```python
from build123d import *

# Parameters (mm, degrees)
F0_W          = 28
F0_H          = 28
F1_DEPTH      = 384.5
F2_W          = 32
F2_H          = 32
F2_W_2        = 28
F2_H_2        = 28
F3_DEPTH      = 608
F3_DEPTH_BACK = 25
F4_W          = 99.2901008725
F4_H          = 100
F5_DEPTH      = 6
F6_R          = 41
F7_DEPTH      = 32.001


with BuildPart() as f1:
    # F0 (on Right) → F1 (new body, symmetric)
    with BuildSketch(Plane.YZ):
        with BuildLine():
            ThreePointArc((-335, -14), (-334.4142135624, -15.4142135624), (-333, -16))
            Line((-333, -16), (-305, -16))
            ThreePointArc((-305, -16), (-303.5857864376, -15.4142135624), (-303, -14))
            Line((-303, -14), (-303, 14))
            ThreePointArc((-303, 14), (-303.5857864376, 15.4142135624), (-305, 16))
            Line((-305, 16), (-333, 16))
            ThreePointArc((-333, 16), (-334.4142135624, 15.4142135624), (-335, 14))
            Line((-335, 14), (-335, -14))
        make_face()
        with Locations((-319, 0)):
            Rectangle(F0_W, F0_H, mode=Mode.SUBTRACT)
    extrude(amount=F1_DEPTH, both=True)



with BuildPart() as f1b:
    # F0 (on Right) → F1, piece 2 (new body, symmetric)
    with BuildSketch(Plane.YZ):
        with BuildLine():
            ThreePointArc((335, 14), (334.4142135624, 15.4142135624), (333, 16))
            Line((333, 16), (305, 16))
            ThreePointArc((305, 16), (303.5857864376, 15.4142135624), (303, 14))
            Line((303, 14), (303, -14))
            ThreePointArc((303, -14), (303.5857864376, -15.4142135624), (305, -16))
            Line((305, -16), (333, -16))
            ThreePointArc((333, -16), (334.4142135624, -15.4142135624), (335, -14))
            Line((335, -14), (335, 14))
        make_face()
        with Locations((319, 0)):
            Rectangle(F0_W, F0_H, mode=Mode.SUBTRACT)
    extrude(amount=F1_DEPTH, both=True)


with BuildPart() as f1_1:
    add(f1.part)

    add(f1b.part)  # F3 merges F1b
    # F2 (on face) → F3 (join, two sides)
    with BuildSketch(Plane(origin=(0, -303, 0), x_dir=(-1, 0, 0), z_dir=(0, 1, 0))) as f3_sk:
        with Locations((-65.2901008725, 0)):
            Rectangle(F2_W, F2_H)
        with Locations((-65.2901008725, 0)):
            Rectangle(F2_W_2, F2_H_2, mode=Mode.SUBTRACT)
        with Locations((65.2901008725, 0)):
            Rectangle(F2_W, F2_H)
        with Locations((65.2901008725, 0)):
            Rectangle(F2_W_2, F2_H_2, mode=Mode.SUBTRACT)
    extrude(amount=F3_DEPTH)
    extrude(f3_sk.sketch, amount=-F3_DEPTH_BACK)

    # F4 (on face) → F5 (join)
    with BuildSketch(Plane.XY.offset(16)):
        with Locations((0.3549495637, 0)):
            Rectangle(F4_W, F4_H)
    extrude(amount=-F5_DEPTH)

    # F6 (on face) → F7 (cut, through all)
    with BuildSketch(Plane.XY.offset(16)):
        Circle(F6_R)
    extrude(amount=-F7_DEPTH, mode=Mode.SUBTRACT)


solid = f1_1.part
```
Input: part model. Units: mm. Frame: model coordinates. A direction names the side the tool comes from. Round coordinates to 2 decimals unless told otherwise and drop trailing zeros. Write each loop counter-clockwise with the first axis right and the second up, starting at its lowest first coordinate (ties: lowest second). Pieces come first, ordered by that corner, then holes. Notation, with made-up numbers: (-34, 18) - (13, 18) arc R20 cw to (13, 47) - close; hole circle Ø7 at (43.25, 3). An arc over 180 degrees is marked (long way). Write item = value, one per line.
(1) Section query B-B on x = -191.5. Output: boundary loops of the cut face in (y, z).
Geometry check:
outline = (-335, -14) arc R2 ccw to (-333, -16) - (-305, -16) arc R2 ccw to (-303, -14) - (-303, 14) arc R2 ccw to (-305, 16) - (-333, 16) arc R2 ccw to (-335, 14) - close; (303, -14) arc R2 ccw to (305, -16) - (333, -16) arc R2 ccw to (335, -14) - (335, 14) arc R2 ccw to (333, 16) - (305, 16) arc R2 ccw to (303, 14) - close; hole (-333, -14) - (-305, -14) - (-305, 14) - (-333, 14) - close; hole (305, -14) - (333, -14) - (333, 14) - (305, 14) - close
(2) Access query for faces 1 (the flat face through (1, 303, 0)), 2 (the flat face through (81.29, -316, 0)), 3 (the flat face through (51.29, -4, 0)), 4 (the flat face through (5, 319, -14)). Directions: +Z, -Z, +X, -X, +Y, -Y. A direction counts if a zero-diameter tool reaches every point of the face in a straight line with its end or side. Return the directions, or none.
Geometry check:
face_1 = +Z, -Z
face_2 = +X
face_3 = none
face_4 = +X, -X
(3) Section query C-C on x = 0. State how many separate pieces and enclosed holes the cut face has, then the cut area to 3 significant figures.
Geometry check:
separate_pieces = 4
enclosed_holes = 2
area = 581 mm^2
(4) Material intervals for probe 1 along X at (y, z) = (-117, 11.5); probe 2 along Y at (x, z) = (227, 1.5); probe 3 along Y at (x, z) = (0, 11.65), sorted ascending.
Geometry check:
probe_1 = -81.29 to -79.29, -51.29 to -49.29, 49.29 to 51.29, 79.29 to 81.29
probe_2 = -335 to -333, -305 to -303, 303 to 305, 333 to 335
probe_3 = -335 to -333, -305 to -303, -50 to -41, 41 to 50, 303 to 305, 333 to 335
(5) Contact query for flat-ended pins moving along their axis: pin 1 Ø1.5 at (y, z) = (-211.5, 7) entering from -X; pin 2 Ø6 at (y, z) = (-30.5, 2.5) entering from +X. Output: stop coordinate, or through.
Geometry check:
pin_1 = -81.29
pin_2 = 81.29
(6) Pull-direction query (Y, two-part tool) for faces 5 (the flat face through (-384.5, -317.89, -14.15)), 6 (the flat face through (-51.29, -316, 0)); classes: +Y half, -Y half, draft (parallel to the pull), parting line (faces both ways), or undercut.
Geometry check:
face_5 = draft
face_6 = undercut
(7) Section query A-A on y = 150.5. Output: boundary loops of the cut face in (x, z), then the cut area to 3 significant figures.
Geometry check:
outline = (-81.29, -16) - (-49.29, -16) - (-49.29, 16) - (-81.29, 16) - close; (49.29, -16) - (81.29, -16) - (81.29, 16) - (49.29, 16) - close; hole (-79.29, -14) - (-51.29, -14) - (-51.29, 14) - (-79.29, 14) - close; hole (51.29, -14) - (79.29, -14) - (79.29, 14) - (51.29, 14) - close
area = 480 mm^2
